Verification items for the finished model (mm, model axes). A direction names the side the tool comes from. Coordinates: 2 decimals unless noted, no trailing zeros. Write each loop counter-clockwise with the first axis right and the second up, starting at its lowest first coordinate (ties: lowest second). Pieces come first, ordered by that corner, then holes. Notation, with made-up numbers: M 50,76.5 L 100,76.5 A18 ccw 100,103.5 Z; hole C 35.25,-0.75 d8. An arc over 180 degrees is marked long. One line per item, written item: value.
```python
from build123d import *

# Parameters (mm, degrees)
BOSS_EXTRUDE1_DEPTH = 2.5
BOSS_EXTRUDE2_DEPTH = 2.5
SKETCH3_R           = 8
SKETCH3_R_2         = 3
BOSS_EXTRUDE3_DEPTH = 5
SKETCH4_R           = 5.5
CUT_EXTRUDE1_DEPTH  = 5


with BuildPart() as part:
    # Sketch1 → Boss-Extrude1 (new body)
    with BuildSketch(Plane(origin=(0, 0, 0), x_dir=(1, 0, 0), z_dir=(0, 1, 0))):
        with BuildLine():
            ThreePointArc((-18.401121459, 30.941860465), (-31.176914536, 18), (-35.996997933, 0.464908409))
            ThreePointArc((-35.996997933, 0.464908409), (-36.88129594, -2.851352197), (-39.235664305, -5.348654136))
            ThreePointArc((-39.235664305, -5.348654136), (-44.167295593, -25.5), (-24.249902511, -31.304754955))
            ThreePointArc((-24.249902511, -31.304754955), (-20.909991408, -30.51446311), (-17.595876474, -31.406768874))
            ThreePointArc((-17.595876474, -31.406768874), (0, -36), (17.595876474, -31.406768874))
            ThreePointArc((17.595876474, -31.406768874), (20.909991408, -30.51446311), (24.249902511, -31.304754955))
            ThreePointArc((24.249902511, -31.304754955), (44.167295593, -25.5), (39.235664305, -5.348654136))
            ThreePointArc((39.235664305, -5.348654136), (36.88129594, -2.851352197), (35.996997933, 0.464908409))
            ThreePointArc((35.996997933, 0.464908409), (31.176914536, 18), (18.401121459, 30.941860465))
            ThreePointArc((18.401121459, 30.941860465), (15.971304532, 33.365815307), (14.985761794, 36.653409091))
            ThreePointArc((14.985761794, 36.653409091), (0, 51), (-14.985761794, 36.653409091))
            ThreePointArc((-14.985761794, 36.653409091), (-15.971304532, 33.365815307), (-18.401121459, 30.941860465))
        make_face()
    extrude(amount=BOSS_EXTRUDE1_DEPTH)

    # Sketch2 → Boss-Extrude2 (add)
    with BuildSketch(Plane(origin=(0, 2.5, 0), x_dir=(1, 0, 0), z_dir=(0, 1, 0))):
        with BuildLine():
            ThreePointArc((33.49720641, 0.432623103), (34.697325134, -4.068016291), (37.892539344, -7.45721178))
            ThreePointArc((37.892539344, -7.45721178), (42.002232084, -24.25), (25.404404515, -29.087295795))
            ThreePointArc((25.404404515, -29.087295795), (20.871668018, -28.014756864), (16.373940607, -29.225743258))
            ThreePointArc((16.373940607, -29.225743258), (0, -33.5), (-16.373940607, -29.225743258))
            ThreePointArc((-16.373940607, -29.225743258), (-20.871668018, -28.014756864), (-25.404404515, -29.087295795))
            ThreePointArc((-25.404404515, -29.087295795), (-42.002232084, -24.25), (-37.892539344, -7.45721178))
            ThreePointArc((-37.892539344, -7.45721178), (-34.697325134, -4.068016291), (-33.49720641, 0.432623103))
            ThreePointArc((-33.49720641, 0.432623103), (-29.011851027, 16.75), (-17.123265802, 28.793120155))
            ThreePointArc((-17.123265802, 28.793120155), (-13.825657116, 32.082773155), (-12.488134829, 36.544507576))
            ThreePointArc((-12.488134829, 36.544507576), (0, 48.5), (12.488134829, 36.544507576))
            ThreePointArc((12.488134829, 36.544507576), (13.825657116, 32.082773155), (17.123265802, 28.793120155))
            ThreePointArc((17.123265802, 28.793120155), (29.011851027, 16.75), (33.49720641, 0.432623103))
        make_face()
    extrude(amount=BOSS_EXTRUDE2_DEPTH)

    # Sketch3 → Boss-Extrude3 (add)
    with BuildSketch(Plane(origin=(0, 5, 0), x_dir=(1, 0, 0), z_dir=(0, 1, 0))):
        with Locations((0, 36)):
            Circle(SKETCH3_R)
        with Locations((0, 36)):
            Circle(SKETCH3_R_2, mode=Mode.SUBTRACT)
        with Locations((31.176914536, -18)):
            Circle(SKETCH3_R)
        with Locations((31.176914536, -18)):
            Circle(SKETCH3_R_2, mode=Mode.SUBTRACT)
        with Locations((-31.176914536, -18)):
            Circle(SKETCH3_R)
        with Locations((-31.176914536, -18)):
            Circle(SKETCH3_R_2, mode=Mode.SUBTRACT)
    extrude(amount=BOSS_EXTRUDE3_DEPTH)

    # Sketch4 → Cut-Extrude1 (cut)
    with BuildSketch(Plane.XZ):
        with Locations((31.176914536, 18)):
            Circle(SKETCH4_R)
        with Locations((0, -36)):
            Circle(SKETCH4_R)
        with Locations((-31.176914536, 18)):
            Circle(SKETCH4_R)
    extrude(amount=-CUT_EXTRUDE1_DEPTH, mode=Mode.SUBTRACT)


solid = part.part
```
Item 1: Cross-section at B-B, the plane x = 0. Enter the section's corners in (y, z).
The answers:
outline: M 0,-51 L 2.5,-51 L 2.5,-48.5 L 5,-48.5 L 5,-44 L 10,-44 L 10,-39 L 5,-39 L 5,-41.5 L 0,-41.5 Z; M 0,-30.5 L 5,-30.5 L 5,-33 L 10,-33 L 10,-28 L 5,-28 L 5,33.5 L 2.5,33.5 L 2.5,36 L 0,36 Z
Item 2: Go/stop test with flat-tipped pins: P1, Ø4, axis at y = 8, z = 13.5, coming from the -X side; P2, Ø8, axis at x = 0, z = -36, coming from the -Y side; P3, Ø6, axis at y = 1.5, z = 1, coming from the -X side; P4, Ø1, axis at y = 6.5, z = -25.5, coming from the -X side. Record where each tip stops, or that it passes through.
The answers:
P1: stops at x = -38.78
P2: stops at y = 5
P3: stops at x = -37.68
P4: passes through
Item 3: Cross-section at C-C, the plane y = 6.5. Enter the section's corners in (x, z).
The answers:
outline: C -31.18,18 d16; C 0,-36 d16; C 31.18,18 d16; hole C -31.18,18 d6; hole C 0,-36 d6; hole C 31.18,18 d6
Item 4: Cross-section at A-A, the plane z = 18. Give the number of separate pieces and of enclosed holes in the cut face, and give its area (3 significant figures).
The answers:
separate pieces: 3
enclosed holes: 0
area: 439 mm²
Item 5: Scan lines: line 1 (X direction, y = 8.4, z = 18); line 2 (X direction, y = 1, z = 14); line 3 (Z direction, x = 4, y = 3.25). Record each from-to range of solid material in increasing order.
The answers:
line 1: x = -39.18 to -34.18, -28.18 to -23.18, 23.18 to 28.18, 34.18 to 39.18
line 2: x = -45.63 to -34.95, -27.4 to 27.4, 34.95 to 45.63
line 3: z = -47.84 to -39.77, -32.23 to 33.26
Item 6: Access from +Z, -Z, +X, -X, +Y, -Y to the whole of each face (thin tool, end or side, straight path). Record for faces 1 (the face through (-13.86, 3.732, -32.026)), 2 (the face through (-20.806, 3.732, 28.016)), 3 (the face through (13.5, 2.5, 31)), 4 (the face through (34, 5, 16)), 5 (the face through (-0.267, 3.732, -48.497)).
The answers:
face 1: -Z, -X, +Y
face 2: +Z, +Y
face 3: +Y
face 4: -Y
face 5: -Z, +Y
Item 7: Draft check along Z on faces 6 (the face through (-37.5, 7.5, 22.9)), 7 (the face through (33.948, 7.465, 19.149)), 8 (the face through (31.305, 1.232, -17.777)). Enter one of: released by +Z, released by -Z, zero draft, split by the parting line, or undercut.
The answers:
face 6: split by the parting line
face 7: undercut
face 8: released by -Z
